CAD build for the part. Positions are in the model's coordinates, mm. A direction names the side the tool comes from. Round coordinates to 2 decimals unless told otherwise and drop trailing zeros. Loops run counter-clockwise (first coordinate to the right, second up) from the corner with the lowest first, then second, coordinate; pieces in that order, holes last. Notation, with made-up numbers: (31.5, 28.25) - (58.5, 28.25) arc R21 cw to (58.5, 38.25) - close; hole circle Ø1 at (18.25, 76.25). An arc over 180 degrees is marked (long way). One line per question, with ' | ' between items.
```python
from build123d import *

# Parameters (mm, degrees)
F1_DEPTH     = 25.4
F2_SIZE      = 12.69999
F3_T1_DEPTH  = 188.8441409877
F4_DEPTH     = 20.574
F5_T1_DEPTH  = 49.2316398108
F5_T3_DEPTH  = 43.3636113916
F5_T5_DEPTH  = 43.3636113916
F5_T7_DEPTH  = 60.6732038629
F5_T12_DEPTH = 43.5108377847
F5_T17_DEPTH = 43.5108377847
F5_T22_DEPTH = 43.5108377847
F5_T27_DEPTH = 43.5108377847


# Not quite as in the source:
# - a fillet or chamfer that OpenCascade refuses, or shapes differently, is made with other operations: its cross-section is extruded or revolved along the edge and cut away or added
# - a fillet or chamfer is up to 0.001 mm smaller than in the source, because OpenCascade refuses the exact size


with BuildPart() as f1:
    # F0 (on Top) → F1 (new body)
    with BuildSketch(Plane.XY):
        Polygon((-6.9792079739, 0), (0, 0), (6.9792079739, 0), (13.9584159479, 0), (0, 76.0870501399), (-11.1239045018, 136.72323427), (-13.9584159479, 152.1741002798), (-13.9584159479, 76.0870501399), (-13.9584159479, 0), align=None)
        Polygon((6.9792079739, 0), (0, 0), (-6.9792079739, 0), (-6.9792079739, -30.6587181985), (-4.935038276, -30.6587181985), (6.9792079739, -30.6587181985), align=None)
    extrude(amount=F1_DEPTH)

    # F2 (size 12.7 in the source; OpenCascade refuses exactly that, so slightly less here)
    f2_edges = [f1.edges().sort_by_distance(p)[0] for p in [
        (-13.958416, 76.08705, 25.4),
        (-13.958416, 76.08705, 0),
    ]]
    chamfer(f2_edges, length=F2_SIZE)

    # F3: chamfer of 10.16 on 2 edges, made by hand

    # F3_s2 → F3_t1 (cut)
    with BuildSketch(Plane(origin=(5.1691181491, -28.1767611209, 0), x_dir=(0, 0, 1), z_dir=(-0.1804419719, 0.9835856316, 0))):
        Polygon((15.24, 13.7292973667), (25.4, 3.5692973667), (25.4, 13.7292973667), align=None)
        Polygon((10.16, 13.7292973667), (0, 3.5692973667), (0, 13.7292973667), align=None)
    extrude(amount=F3_T1_DEPTH, mode=Mode.SUBTRACT)

    # F4 (add): a face of the model
    f4_faces = [f1.faces().sort_by_distance(p)[0] for p in [
        (0.5158291465, -30.6587181985, 12.7),
    ]]
    extrude(f4_faces, amount=F4_DEPTH)

    # F5: chamfer of 6.858 on 6 edges, made by hand

    # F5_s2 → F5_t1 (cut)
    with BuildSketch(Plane.XY.offset(-11.9158199054)):
        Polygon((-0.1212079739, -51.2327181985), (-6.9792079739, -44.3747181985), (-6.9792079739, -51.2327181985), align=None)
    extrude(amount=F5_T1_DEPTH, mode=Mode.SUBTRACT)

    # F5_s4 → F5_t3 (cut)
    with BuildSketch(Plane(origin=(-18.8209558228, 0, 18.8209558228), x_dir=(0, 1, 0), z_dir=(0.7071067812, 0, -0.7071067812))):
        Polygon((-51.2327181985, 5.9681584787), (-44.3747181985, -0.8898415213), (-51.2327181985, -0.8898415213), align=None)
    extrude(amount=F5_T3_DEPTH, mode=Mode.SUBTRACT)

    # F5_s6 → F5_t5 (cut)
    with BuildSketch(Plane(origin=(-6.1209558228, 0, -6.1209558228), x_dir=(0, 1, 0), z_dir=(0.7071067812, 0, 0.7071067812))):
        Polygon((-51.2327181985, 11.9923537635), (-44.3747181985, 18.8503537635), (-51.2327181985, 18.8503537635), align=None)
    extrude(amount=F5_T5_DEPTH, mode=Mode.SUBTRACT)

    # F5_s8 → F5_t7 (cut)
    with BuildSketch(Plane.XY.offset(-17.6366019315)):
        Polygon((0.1212079739, -51.2327181985), (6.9792079739, -44.3747181985), (6.9792079739, -51.2327181985), align=None)
    extrude(amount=F5_T7_DEPTH, mode=Mode.SUBTRACT)


with BuildPart() as f5_tool10:
    # F5_s11 → F5_t12 (new body)
    with BuildSketch(Plane.YZ.offset(-18.8950278793)):
        Polygon((-51.2327181985, 6.858), (-44.3747181985, 0), (-51.2327181985, 0), align=None)
    extrude(amount=F5_T12_DEPTH)

    split(bisect_by=Plane(origin=(-16.0034385627, -22.6322798599, -16.0034385627), x_dir=(0.8164965809, -0.5773502692, 0), z_dir=(-0.5, -0.7071067812, -0.5)), keep=Keep.TOP)


with BuildPart() as f1_1:
    add(f1.part)

    # F5_t9: cut F5_tool10
    add(f5_tool10.part, mode=Mode.SUBTRACT)


with BuildPart() as f5_tool15:
    # F5_s16 → F5_t17 (new body)
    with BuildSketch(Plane.YZ.offset(-18.8950278793)):
        Polygon((-51.2327181985, 6.858), (-44.3747181985, 0), (-51.2327181985, 0), align=None)
    extrude(amount=F5_T17_DEPTH)

    split(bisect_by=Plane(origin=(25.6769630862, -25.6769630862, 0), x_dir=(0, 0, 1), z_dir=(0.7071067812, -0.7071067812, 0)), keep=Keep.TOP)


with BuildPart() as f1_2:
    add(f1_1.part)

    # F5_t14: cut F5_tool15
    add(f5_tool15.part, mode=Mode.SUBTRACT)


with BuildPart() as f5_tool20:
    # F5_s21 → F5_t22 (new body)
    with BuildSketch(Plane.YZ.offset(-18.8950278793)):
        Polygon((-44.3747181985, 25.4), (-51.2327181985, 18.542), (-51.2327181985, 25.4), align=None)
    extrude(amount=F5_T22_DEPTH)

    split(bisect_by=Plane(origin=(-22.3534385627, -31.612535981, 22.3534385627), x_dir=(0.8164965809, -0.5773502692, 0), z_dir=(-0.5, -0.7071067812, 0.5)), keep=Keep.TOP)


with BuildPart() as f1_3:
    add(f1_2.part)

    # F5_t19: cut F5_tool20
    add(f5_tool20.part, mode=Mode.SUBTRACT)


with BuildPart() as f5_tool25:
    # F5_s26 → F5_t27 (new body)
    with BuildSketch(Plane.YZ.offset(-18.8950278793)):
        Polygon((-44.3747181985, 25.4), (-51.2327181985, 18.542), (-51.2327181985, 25.4), align=None)
    extrude(amount=F5_T27_DEPTH)

    split(bisect_by=Plane(origin=(25.6769630862, -25.6769630862, 0), x_dir=(0, 0, 1), z_dir=(0.7071067812, -0.7071067812, 0)), keep=Keep.TOP)


with BuildPart() as f1_4:
    add(f1_3.part)

    # F5_t24: cut F5_tool25
    add(f5_tool25.part, mode=Mode.SUBTRACT)


solid = f1_4.part
```
(1) Drop flat-ended pins along their axis: P1, Ø1.5, axis at x = -7.5, z = 19.5, coming from the -Y side; P2, Ø5, axis at x = -5.5, z = 10, coming from the -Y side; P3, Ø8, axis at x = -4, y = 65, coming from the -Z side. Give the stop position or say it passes through.
Results found:
P1: stops at y = -44.6 | P2: stops at y = -48.35 | P3: stops at z = 3.13
(2) Tool access for faces 1 (the face through (-6.979, -22, 13)), 2 (the face through (-1.05, -47.09, 21.77)), 3 (the face through (6.979, -22, 13)): list every direction of +Z, -Z, +X, -X, +Y, -Y with a clear straight run to the whole face (end or side of a thin tool).
Results found:
face 1: +Z, -Z, -X, -Y | face 2: +Z, -X, -Y | face 3: +Z, -Z, +X, -Y
(3) Cut at A-A, the plane y = -25.5. Write the cut outline in (x, z).
Results found:
outline: (-6.98, 5.72) - (-1.26, 0) - (6.98, 0) - (6.98, 25.4) - (-1.26, 25.4) - (-6.98, 19.68) - close
(4) Probe L1, parallel to Z at x = -1.5, y = 11; L2, parallel to Z at x = -11, y = 42.5; L3, parallel to X at y = 119.5, z = 13.5. List the from-to ranges inside material, lowest first.
Results found:
L1: z = 0.24 to 25.16 | L2: z = 9.74 to 15.66 | L3: x = -13.16 to -7.96
